Design review of the part built by this model. Coordinates are the model's own, in mm. A direction names the side the tool comes from. Coordinates: 2 decimals unless noted, no trailing zeros. Loops run counter-clockwise (first coordinate to the right, second up) from the corner with the lowest first, then second, coordinate; pieces in that order, holes last. Notation, with made-up numbers: M 1.5,-21 L 42.5,-21 A10 ccw 42.5,-4 Z; hole C 52,42 d6. An arc over 180 degrees is marked long. Answer as CSV lines item,"result". Start each with the question number.
from build123d import *

# Parameters (mm, degrees)
F0_W     = 50
F0_H     = 30
F1_DEPTH = 50
F3_DEPTH = 20
F4_DEPTH = 50.001
F6_DEPTH = 25
F8_DEPTH = 20


with BuildPart() as f1:
    # F0 (on Top) → F1 (new body)
    with BuildSketch(Plane.XY):
        Rectangle(F0_W, F0_H)
    extrude(amount=F1_DEPTH)

    # F2 (on face) → F3 (cut)
    with BuildSketch(Plane.XY.offset(50)):
        Polygon((-25, -15), (-15, -15), (-15, -10), (15, -10), (15, -15), (25, -15), (25, -5), (-25, -5), align=None)
    extrude(amount=-F3_DEPTH, mode=Mode.SUBTRACT)

    # F4 (cut, through all): a face of the model
    f4_faces = [f1.faces().sort_by_distance(p)[0] for p in [
        (0, -12.5, 50),
    ]]
    extrude(f4_faces, amount=-F4_DEPTH, mode=Mode.SUBTRACT)

    # F5 (on face) → F6 (cut)
    with BuildSketch(Plane(origin=(0, 0, 0), x_dir=(1, 0, 0), z_dir=(0, 0, -1))):
        Polygon((-25, 15), (-25, 5), (25, 5), (25, 15), (15, 15), (15, 10), (-15, 10), (-15, 15), align=None)
    extrude(amount=-F6_DEPTH, mode=Mode.SUBTRACT)

    # F7 (on face) → F8 (cut)
    with BuildSketch(Plane(origin=(0, 15, 0), x_dir=(-1, 0, 0), z_dir=(0, 1, 0))):
        Polygon((-4.6503130347, 33.1786386669), (-4.6503130347, 28.1786386669), (4.6503130347, 28.1786386669), (4.6503130347, 33.1786386669), (20, 50), (-20, 50), align=None)
    extrude(amount=-F8_DEPTH, mode=Mode.SUBTRACT)


solid = f1.part
Item 1: For line 1 along X through (y, z) = (8.5, 30.5); line 2 along Y through (x, z) = (20, 46.5); line 3 along Y through (x, z) = (0, 29), list the stretches that pass through material, from the lowest coordinate up. Write a range as from..to.
Item 2: Add section D-D (z = 29). Give the boundary of the cut face in (x, y), plus the area to 3 significant figures.
Item 3: Mouldability with a two-part tool opening along X and no side actions: class faces 4 (the face through (25, 3, 25)), 5 (the face through (0, -10, 28)), 6 (the face through (0, -5, 12)) as released by +X, released by -X, zero draft, split by the parting line, or undercut.
Item 4: For pin 1 (6 mm diameter, centred on x = 15, z = 35, fed in from -Y); pin 2 (10 mm diameter, centred on y = -7, z = 22, fed in from +X); pin 3 (4.5 mm diameter, centred on x = 2, y = 7, fed in from +Z); pin 4 (2 mm diameter, centred on x = 4, y = -8.5, fed in from +Z), all flat-tipped, find the tip position at first contact; note any pin that passes through.
Item 5: Add section C-C (x = -2). Give the boundary of the cut face in (y, z).
Item 6: For faces 1 (the face through (0, 5, 28.179)), 2 (the face through (15, -12, 28)), 3 (the face through (17, -5, 38)), list the 3-axis set-ups (+Z, -Z, +X, -X, +Y, -Y) from which the entire face can be reached by the end or side of a thin tool; tool diameter is ignored.
Item 7: Add section B-B (z = 37). Give the boundary of the cut face in (x, y).
Item 8: Add section A-A (y = -13). Give the boundary of the cut face in (x, z).
Response:
1,line 1,"-25..-4.65, 4.65..25"
1,line 2,"-5..15"
1,line 3,"-10..-5"
2,outline,"M -25,-15 L -15,-15 L -15,-10 L 15,-10 L 15,-15 L 25,-15 L 25,15 L 4.65,15 L 4.65,-5 L -4.65,-5 L -4.65,15 L -25,15 Z"
2,area,"1,160 mm²"
3,face 4,"released by +X"
3,face 5,"undercut"
3,face 6,"zero draft"
4,pin 1,"y = -5"
4,pin 2,"x = 25"
4,pin 3,"z = 28.18"
4,pin 4,"z = 30"
5,outline,"M -10,25 L -5,25 L -5,0 L 15,0 L 15,28.18 L -5,28.18 L -5,30 L -10,30 Z"
6,face 1,"+Z, +Y"
6,face 2,"+Z, -Z, -Y"
6,face 3,"+Z, +X, -X, -Y"
7,outline,"M -25,-5 L -8.14,-5 L -8.14,15 L -25,15 Z; M 8.14,-5 L 25,-5 L 25,15 L 8.14,15 Z"
8,outline,"M -25,25 L -15,25 L -15,30 L -25,30 Z; M 15,25 L 25,25 L 25,30 L 15,30 Z"
